Check sheet for the modelled part. Datum: model origin and axes. Units: mm. Give positions to 0.01 mm unless a question says otherwise; leave off trailing zeros. Order: outer loops, then holes, each group sorted by start corner. A loop starts at its lowest first (then second) coordinate and runs counter-clockwise, first axis right, second up. Notation, with made-up numbers: M -3,35.25 L 11,35.25 A31 cw 11,63.25 Z; hole C 84,-40 d11. An arc over 180 degrees is marked long. Answer in a Markdown table with one row per item. Add a question column.
Autodesk Fusion 360 part; units mm, degrees
sketch "Sketch1" plane through (0, 0, 0) normal (0, 0, 1) x (1, 0, 0)
  line L0 (-84.9, 11.9) -> (84.9, 11.9)
  line L1 (84.9, 11.9) -> (84.9, -11.9)
  line L2 (84.9, -11.9) -> (-84.9, -11.9)
  line L3 (-84.9, -11.9) -> (-84.9, 11.9)
  circle A0 centre (-81.9, 8.9) radius 3
  circle A1 centre (-81.9, -8.9) radius 3
  circle A2 centre (81.9, 8.9) radius 3
  circle A3 centre (81.9, -8.9) radius 3
  line L4 (-107.1873, 0) -> (-105, 0)
  line L5 (-105, 0) -> (105, 0) construction
  circle A4 centre (-81, 0) radius 2.2
  circle A5 centre (81, 0) radius 2.2
  dimension "d21" = 169.8
  dimension "d22" = 84.9
  dimension "d23" = 23.8
  dimension "d24" = 11.9
  dimension "d25" = 6
  dimension "d26" = 6
  dimension "d27" = 6
  dimension "d28" = 6
  dimension "d29" = 210
  dimension "d30" = 4.4
  dimension "d31" = 4.4
  dimension "d32" = 3.9
  dimension "d33" = 3.9
extrude "Extrude1" add sketch "Sketch1" along normal blind 2.8 contours L0 L1 L2 L3 A0 A1 A2 A3 | A0 | A2 | A1 | A3
sketch "Sketch2" plane through (0, 0, 2.8) normal (0, 0, 1) x (-1, 0, 0)
  circle A0 centre (81, 0) radius 2.2
  circle A1 centre (-81, 0) radius 2.2
  arc A2 (81.9, -11.9) -> (84.9, -8.9) centre (81.9, -8.9) ccw
  line L0 (84.9, -8.9) -> (84.9, 8.9)
  arc A3 (84.9, 8.9) -> (81.9, 11.9) centre (81.9, 8.9) ccw
  line L1 (81.9, 11.9) -> (-81.9, 11.9)
  arc A4 (-81.9, 11.9) -> (-84.9, 8.9) centre (-81.9, 8.9) ccw
  line L2 (-84.9, 8.9) -> (-84.9, -8.9)
  arc A5 (-84.9, -8.9) -> (-81.9, -11.9) centre (-81.9, -8.9) ccw
  line L3 (-81.9, -11.9) -> (81.9, -11.9)
  line L4 (-81.9, -13.3) -> (81.9, -13.3)
  arc A6 (81.9, -13.3) -> (86.3, -8.9) centre (81.9, -8.9) ccw
  line L5 (86.3, -8.9) -> (86.3, 8.9)
  arc A7 (86.3, 8.9) -> (81.9, 13.3) centre (81.9, 8.9) ccw
  line L6 (81.9, 13.3) -> (-81.9, 13.3)
  arc A8 (-81.9, 13.3) -> (-86.3, 8.9) centre (-81.9, 8.9) ccw
  line L7 (-86.3, 8.9) -> (-86.3, -8.9)
  arc A9 (-86.3, -8.9) -> (-81.9, -13.3) centre (-81.9, -8.9) ccw
  dimension "d36" = 1.4
extrude "Extrude2" add sketch "Sketch2" along normal blind 2.4 contours A2 L0 A3 L1 A4 L2 A5 L3 | L4 A6 L5 A7 L6 A8 L7 A9
chamfer "Chamfer1" distance 0.6 angle 45 8 edges at (86.3, 0, 5.2) (85.0113, 12.0113, 5.2) (0, 13.3, 5.2) (-85.0113, 12.0113, 5.2) (-86.3, 0, 5.2) (-85.0113, -12.0113, 5.2) (0, -13.3, 5.2) (85.0113, -12.0113, 5.2)
sketch "Sketch4" plane through (-1.7827, -2.3697, 0) normal (0, 0, -1) x (1, 0, 0)
  circle A0 centre (-79.2173, -2.3697) radius 2.2
  circle A1 centre (82.7827, -2.3697) radius 2.2
  arc A2 (-83.1173, -11.2697) -> (-80.1173, -14.2697) centre (-80.1173, -11.2697) ccw
  line L0 (-80.1173, -14.2697) -> (83.6827, -14.2697)
  arc A3 (83.6827, -14.2697) -> (86.6827, -11.2697) centre (83.6827, -11.2697) ccw
  line L1 (86.6827, -11.2697) -> (86.6827, 6.5303)
  arc A4 (86.6827, 6.5303) -> (83.6827, 9.5303) centre (83.6827, 6.5303) ccw
  line L2 (83.6827, 9.5303) -> (-80.1173, 9.5303)
  arc A5 (-80.1173, 9.5303) -> (-83.1173, 6.5303) centre (-80.1173, 6.5303) ccw
  line L3 (-83.1173, 6.5303) -> (-83.1173, -11.2697)
  line L4 (-82.6173, 6.5303) -> (-82.6173, -11.2697)
  arc A6 (-82.6173, -11.2697) -> (-80.1173, -13.7697) centre (-80.1173, -11.2697) ccw
  line L5 (-80.1173, -13.7697) -> (83.6827, -13.7697)
  arc A7 (83.6827, -13.7697) -> (86.1827, -11.2697) centre (83.6827, -11.2697) ccw
  line L6 (86.1827, -11.2697) -> (86.1827, 6.5303)
  arc A8 (86.1827, 6.5303) -> (83.6827, 9.0303) centre (83.6827, 6.5303) ccw
  line L7 (83.6827, 9.0303) -> (-80.1173, 9.0303)
  arc A9 (-80.1173, 9.0303) -> (-82.6173, 6.5303) centre (-80.1173, 6.5303) ccw
  dimension "d44" = -0.5
extrude "Extrude4" cut sketch "Sketch4" against normal up to surface (2.8 mm away) contours A2 L0 A3 L1 A4 L2 A5 L3
equation "d22 = d21 / 2"
equation "d24 = d23 / 2"
equation "d26 = d25"
equation "d27 = d25"
equation "d28 = d25"
equation "d33 = d32"
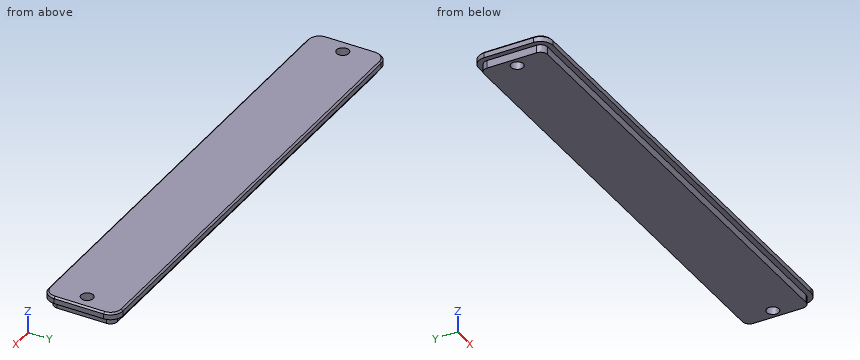
Q1. Thickness scan on probe 1 along X at (y, z) = (0, 3.85); probe 2 along X at (y, z) = (0, 1.5); probe 3 along Y at (x, z) = (81, 2.7). Record the ranges inside material, lowest first.
Q2. Go/stop test with flat-tipped pins: pin 1 (1.4 mm diameter, centred on y = 3.5, z = 1, fed in from -X); pin 2 (1.4 mm diameter, centred on y = 2, z = 2, fed in from +X); pin 3 (3 mm diameter, centred on x = -1, z = 1, fed in from -Y). Record where each tip stops, or that it passes through.
Q3. Cross-section at A-A (z = 1.6). Record the boundary of the cut face in (x, y), and give its area (3 significant figures).
Q4. Cross-section at B-B (x = -6). Record the boundary of the cut face in (y, z), and give its area (3 significant figures).
Values follow:
| question | item | result |
|---|---|---|
| 1 | probe 1 | -86.3 to -83.2, -78.8 to 78.8, 83.2 to 86.3 |
| 1 | probe 2 | -84.4 to -83.2, -78.8 to 78.8, 83.2 to 84.4 |
| 1 | probe 3 | -11.4 to -2.2, 2.2 to 11.4 |
| 2 | pin 1 | x = -84.4 |
| 2 | pin 2 | x = 84.4 |
| 2 | pin 3 | y = -11.4 |
| 3 | outline | M -84.4,-8.9 A2.5 ccw -81.9,-11.4 L 81.9,-11.4 A2.5 ccw 84.4,-8.9 L 84.4,8.9 A2.5 ccw 81.9,11.4 L -81.9,11.4 A2.5 ccw -84.4,8.9 Z; hole C -81,0 d4.4; hole C 81,0 d4.4 |
| 3 | area | 3,810 mm² |
| 4 | outline | M -13.3,2.8 L -11.4,2.8 L -11.4,0 L 11.4,0 L 11.4,2.8 L 13.3,2.8 L 13.3,4.6 L 12.7,5.2 L -12.7,5.2 L -13.3,4.6 Z |
| 4 | area | 127 mm² |
